```python
from build123d import *

# Parameters (mm, degrees)
SKETCH_1_R      = 8
SKETCH_1_R_2    = 5
EXTRUDE_1_DEPTH = 5
SKETCH_4_R      = 16
SKETCH_4_R_2    = 8
EXTRUDE_2_DEPTH = 3
SKETCH_5_R      = 16
SKETCH_5_R_2    = 12.5
EXTRUDE_3_DEPTH = 3
ST2_9_1_D       = 2.9


with BuildPart() as part:
    # 草图1 → 凸台-拉伸1 (new body)
    with BuildSketch(Plane(origin=(0, 0, 606.712583837), x_dir=(-1, 0, 0), z_dir=(0, 0, -1))):
        with Locations((-4.295303519, -1.225452996)):
            Circle(SKETCH_1_R)
        with Locations((-4.295303519, -1.225452996)):
            Circle(SKETCH_1_R_2, mode=Mode.SUBTRACT)
    extrude(amount=EXTRUDE_1_DEPTH)

    # 草图4 → 凸台-拉伸2 (add)
    with BuildSketch(Plane(origin=(0, 0, 606.712583837), x_dir=(-1, 0, 0), z_dir=(0, 0, -1))):
        with Locations((-4.295303519, -1.225452996)):
            Circle(SKETCH_4_R)
        with Locations((-4.295303519, -1.225452996)):
            Circle(SKETCH_4_R_2, mode=Mode.SUBTRACT)
    extrude(amount=EXTRUDE_2_DEPTH)

    # 草图5 → 凸台-拉伸3 (add)
    with BuildSketch(Plane(origin=(0, 0, 603.712583837), x_dir=(-1, 0, 0), z_dir=(0, 0, -1))):
        with Locations((-4.295303519, -1.225452996)):
            Circle(SKETCH_5_R)
        with Locations((-4.295303519, -1.225452996)):
            Circle(SKETCH_5_R_2, mode=Mode.SUBTRACT)
    extrude(amount=-EXTRUDE_3_DEPTH)

    # ST2.9 间隙孔1 (through all)
    with Locations(Plane(origin=(0, 0, 603.712583837), x_dir=(-1, 0, 0), z_dir=(0, 0, -1))):
        with Locations((-4.295303519, 9.774547004), (6.704696481, -1.225452996), (-4.295303519, -12.225452996), (-15.295303519, -1.225452996)):
            Hole(ST2_9_1_D / 2)


solid = part.part
```
Geometry check sheet. Reference: the model listing, model coordinates, mm. A direction names the side the tool comes from. Give positions to 0.01 mm unless a question says otherwise; leave off trailing zeros. Order: outer loops, then holes, each group sorted by start corner. A loop starts at its lowest first (then second) coordinate and runs counter-clockwise, first axis right, second up. Notation, with made-up numbers: (58, 23) - (113, 23) arc R25 ccw to (113, 52) - close; hole circle Ø6 at (12.5, -21.75). An arc over 180 degrees is marked (long way). Answer in a Markdown table with one row per item. Add a question column.
Q1. Cross-section at C-C, the plane z = 605.95. Enter the section's corners in (x, y), then the cut area to 3 significant figures.
Q2. Material ranges on probe 1 along X at (y, z) = (-1.5, 602.2); probe 2 along Y at (x, z) = (7.5, 602.5); probe 3 along Z at (x, y) = (-3.5, 7), recorded low to high. Write a range as from..to.
Q3. Cross-section at D-D, the plane x = -1.5. Enter the section's corners in (y, z).
Q4. Mould release check, pull along Y, two halves, no side actions. Record for faces 1 (the flat face through (12, -5, 603.713)), 2 (the cylindrical face through (16.68, -0.79, 605.23)), 3 (the cylindrical face through (-10.485, -7.354, 605.234)), 4 (the cylindrical face through (-0.323, -3.14, 604.248)): pulls with the +Y half, pulls with the -Y half, needs draft (parallel to the pull), parting line crosses it, or undercut.
Q5. Tool access check on faces 5 (the cylindrical face through (10.644, -6.093, 602.727)), 6 (the cylindrical face through (3.98, -13.64, 605.23)). Record the directions out of +Z, -Z, +X, -X, +Y, -Y that give a thin tool (end or side, any length) a straight path to the whole face; none if there is none.
Q6. Gauge pin test, flat ends, axial feed: pin 1 (3.5 mm diameter, centred on x = 4.3, y = -12.23, fed in from -Z); pin 2 (10 mm diameter, centred on x = 15, y = -2, fed in from +Z); pin 3 (1 mm diameter, centred on y = 6, z = 605.5, fed in from -X); pin 4 (1 mm diameter, centred on y = -7, z = 602.5, fed in from -X). Record the tip position at first contact, or that the pin passes through.
Q7. Cross-section at A-A, the plane x = -7.5. Enter the section's corners in (y, z).
Q8. Cross-section at B-B, the plane y = -2. Enter the section's corners in (x, z).
Check values:
| question | item | result |
|---|---|---|
| 1 | outline | circle Ø32 at (4.3, -1.23); hole circle Ø2.9 at (-6.7, -1.23); hole circle Ø10 at (4.3, -1.23); hole circle Ø2.9 at (4.3, -12.23); hole circle Ø2.9 at (4.3, 9.77); hole circle Ø2.9 at (15.3, -1.23) |
| 1 | area | 699 mm^2 |
| 2 | probe 1 | x = -3.7..-0.7, 9.29..12.29 |
| 2 | probe 2 | y = -8.56..-5.06, 2.61..6.1 |
| 2 | probe 3 | z = 603.71..606.71 |
| 3 | outline | (-16.14, 603.71) - (-6.74, 603.71) - (-6.74, 601.71) - (4.29, 601.71) - (4.29, 603.71) - (13.69, 603.71) - (13.69, 606.71) - (-16.14, 606.71) - close |
| 4 | face 1 | needs draft |
| 4 | face 2 | undercut |
| 4 | face 3 | parting line crosses it |
| 4 | face 4 | undercut |
| 5 | face 5 | -Z |
| 5 | face 6 | +Z, -Z |
| 6 | pin 1 | stops at z = 603.71 |
| 6 | pin 2 | stops at z = 606.71 |
| 6 | pin 3 | stops at x = -10.22 |
| 6 | pin 4 | stops at x = -1.72 |
| 7 | outline | (-12.04, 603.71) - (-2.44, 603.71) - (-2.44, 606.71) - (-12.04, 606.71) - close; (-0.01, 603.71) - (9.59, 603.71) - (9.59, 606.71) - (-0.01, 606.71) - close |
| 8 | outline | (-11.69, 603.71) - (-7.93, 603.71) - (-7.93, 606.71) - (-11.69, 606.71) - close; (-5.48, 603.71) - (-3.67, 603.71) - (-3.67, 601.71) - (-0.64, 601.71) - (-0.64, 606.71) - (-5.48, 606.71) - close; (9.23, 601.71) - (12.26, 601.71) - (12.26, 603.71) - (14.07, 603.71) - (14.07, 606.71) - (9.23, 606.71) - close; (16.52, 603.71) - (20.28, 603.71) - (20.28, 606.71) - (16.52, 606.71) - close |
